Verification items for the finished model (mm, model axes). Coordinates: 2 decimals unless noted, no trailing zeros. Loops run counter-clockwise (first coordinate to the right, second up) from the corner with the lowest first, then second, coordinate; pieces in that order, holes last. Notation, with made-up numbers: (38.25, 11) - (50.25, 11) arc R21 ccw to (50.25, 23) - close; hole circle Ø1 at (-9.75, -19). An arc over 180 degrees is marked (long way). One line per item, written item: value. Start each with the question number.
(1) Section check A-A (x = -1.5). Record the boundary of the cut face in (y, z), plus the area to 3 significant figures.
(2) Thickness scan on probe 1 along X at (y, z) = (18, -39.85); probe 2 along X at (y, z) = (-31.5, -39.7); probe 3 along Y at (x, z) = (-14.5, -39.3). Record the ranges inside material, lowest first. Write a range as [from, to].
(3) Gauge pin test, flat end, axial feed: P1, Ø2, axis at x = 34.45, y = 5.84, coming from the -Z side. Record the tip position at first contact, or that the pin passes through.
(4) Section check B-B (x = 10). Record the boundary of the cut face in (y, z).
(5) Section check C-C (z = -40.35). Count the separate pieces of the cut face and the enclosed holes in it, plus the area to 3 significant figures.
(6) Draft check along Y on faces 1 (the face through (-45.8, 36.99, -39.93)), 2 (the face through (33.947, 36.589, -39.95)), 3 (the face through (-45.702, -37.605, -39.93)), 4 (the face through (34.62, -17.47, -39.95)). Enter one of: +Y half, -Y half, draft (parallel to the pull), parting line (faces both ways), or undercut.
```python
from build123d import *

# Parameters (mm, degrees)
EXTRUDE_1_DEPTH     = 1.5
SKETCH_3_R          = 1.3
CUT_EXTRUDE_1_DEPTH = 65.139634718
CUT_EXTRUDE_2_REACH = 66.14
SKETCH_4_R          = 1.3
CUT_EXTRUDE_3_REACH = 66.14
SKETCH_5_W          = 53
SKETCH_5_H          = 6.5
FILLET_1_R          = 1.5
CUT_EXTRUDE_4_REACH = 66.14
SKETCH_7_R          = 1.3
CUT_EXTRUDE_5_REACH = 66.14


with BuildPart() as part:
    # 草图2 → 凸台-拉伸1 (new body)
    with BuildSketch(Plane(origin=(0, 0, -39.19), x_dir=(-1, 0, 0), z_dir=(0, 0, -1))):
        Polygon((-47.34673203, -34.053824425), (-40.342568974, -41.057987481), (42.249104914, -41.057987481), (49.25326797, -34.053824425), (49.25326797, 33.537849463), (42.249104914, 40.542012519), (-40.342568974, 40.542012519), (-47.34673203, 33.537849463), align=None)
    extrude(amount=EXTRUDE_1_DEPTH)

    # 草图3 → 切除-拉伸1 (cut, through all)
    with BuildSketch(Plane(origin=(0, 0, -40.69), x_dir=(-1, 0, 0), z_dir=(0, 0, -1))):
        with Locations((-34.54673203, -38.257987481)):
            Circle(SKETCH_3_R)
        with Locations((36.45326797, -38.257987481)):
            Circle(SKETCH_3_R)
        with Locations((-34.54673203, 37.742012519)):
            Circle(SKETCH_3_R)
        with Locations((36.45326797, 37.742012519)):
            Circle(SKETCH_3_R)
    extrude(amount=-CUT_EXTRUDE_1_DEPTH, mode=Mode.SUBTRACT)

    # 草图4 → 切除-拉伸2 (cut, up to next)
    with BuildSketch(Plane(origin=(0, 0, -40.69), x_dir=(-1, 0, 0), z_dir=(0, 0, -1)), mode=Mode.PRIVATE) as cut_extrude_2_sk1:
        with Locations((23.45326797, -31.293200074)):
            Circle(SKETCH_4_R)
    cut_extrude_2_tool1 = extrude(cut_extrude_2_sk1.sketch, amount=-CUT_EXTRUDE_2_REACH, mode=Mode.PRIVATE) & part.part
    # 草图4 → 切除-拉伸2 (cut, up to next)
    with BuildSketch(Plane(origin=(0, 0, -40.69), x_dir=(-1, 0, 0), z_dir=(0, 0, -1)), mode=Mode.PRIVATE) as cut_extrude_2_sk2:
        with Locations((-34.558299802, -31.293200074)):
            Circle(SKETCH_4_R)
    cut_extrude_2_tool2 = extrude(cut_extrude_2_sk2.sketch, amount=-CUT_EXTRUDE_2_REACH, mode=Mode.PRIVATE) & part.part
    # 草图4 → 切除-拉伸2 (cut, up to next)
    with BuildSketch(Plane(origin=(0, 0, -40.69), x_dir=(-1, 0, 0), z_dir=(0, 0, -1)), mode=Mode.PRIVATE) as cut_extrude_2_sk3:
        with Locations((23.45326797, 17.742012519)):
            Circle(SKETCH_4_R)
    cut_extrude_2_tool3 = extrude(cut_extrude_2_sk3.sketch, amount=-CUT_EXTRUDE_2_REACH, mode=Mode.PRIVATE) & part.part
    # 草图4 → 切除-拉伸2 (cut, up to next)
    with BuildSketch(Plane(origin=(0, 0, -40.69), x_dir=(-1, 0, 0), z_dir=(0, 0, -1)), mode=Mode.PRIVATE) as cut_extrude_2_sk4:
        with Locations((-34.558299802, 17.742012519)):
            Circle(SKETCH_4_R)
    cut_extrude_2_tool4 = extrude(cut_extrude_2_sk4.sketch, amount=-CUT_EXTRUDE_2_REACH, mode=Mode.PRIVATE) & part.part
    add(cut_extrude_2_tool1.solids().sort_by_distance((-23.453268, -31.2932, -40.69))[0], mode=Mode.SUBTRACT)
    add(cut_extrude_2_tool2.solids().sort_by_distance((34.5583, -31.2932, -40.69))[0], mode=Mode.SUBTRACT)
    add(cut_extrude_2_tool3.solids().sort_by_distance((-23.453268, 17.742013, -40.69))[0], mode=Mode.SUBTRACT)
    add(cut_extrude_2_tool4.solids().sort_by_distance((34.5583, 17.742013, -40.69))[0], mode=Mode.SUBTRACT)

    # 草图5 → 切除-拉伸3 (cut, up to next)
    with BuildSketch(Plane(origin=(0, 0, -40.69), x_dir=(-1, 0, 0), z_dir=(0, 0, -1)), mode=Mode.PRIVATE) as cut_extrude_3_sk1:
        with Locations((-5.64673203, 17.992012519)):
            Rectangle(SKETCH_5_W, SKETCH_5_H)
    cut_extrude_3_tool1 = extrude(cut_extrude_3_sk1.sketch, amount=-CUT_EXTRUDE_3_REACH, mode=Mode.PRIVATE) & part.part
    add(cut_extrude_3_tool1.solids().sort_by_distance((5.646732, 17.992013, -40.69))[0], mode=Mode.SUBTRACT)

    # 圆角1
    fillet_1_edges = [part.edges().sort_by_distance(p)[0] for p in [
        (32.14673203, 14.742012519, -39.94),
        (32.14673203, 21.242012519, -39.94),
        (-20.85326797, 21.242012519, -39.94),
        (-20.85326797, 14.742012519, -39.94),
    ]]
    fillet(fillet_1_edges, radius=FILLET_1_R)

    # 草图7 → 切除-拉伸4 (cut, up to next)
    with BuildSketch(Plane(origin=(0, 0, -40.69), x_dir=(-1, 0, 0), z_dir=(0, 0, -1)), mode=Mode.PRIVATE) as cut_extrude_4_sk1:
        with Locations((-34.44673203, 5.842012519)):
            Circle(SKETCH_7_R)
    cut_extrude_4_tool1 = extrude(cut_extrude_4_sk1.sketch, amount=-CUT_EXTRUDE_4_REACH, mode=Mode.PRIVATE) & part.part
    # 草图7 → 切除-拉伸4 (cut, up to next)
    with BuildSketch(Plane(origin=(0, 0, -40.69), x_dir=(-1, 0, 0), z_dir=(0, 0, -1)), mode=Mode.PRIVATE) as cut_extrude_4_sk2:
        with Locations((-34.44673203, -18.757987481)):
            Circle(SKETCH_7_R)
    cut_extrude_4_tool2 = extrude(cut_extrude_4_sk2.sketch, amount=-CUT_EXTRUDE_4_REACH, mode=Mode.PRIVATE) & part.part
    # 草图7 → 切除-拉伸4 (cut, up to next)
    with BuildSketch(Plane(origin=(0, 0, -40.69), x_dir=(-1, 0, 0), z_dir=(0, 0, -1)), mode=Mode.PRIVATE) as cut_extrude_4_sk3:
        with Locations((-9.84673203, 5.842012519)):
            Circle(SKETCH_7_R)
    cut_extrude_4_tool3 = extrude(cut_extrude_4_sk3.sketch, amount=-CUT_EXTRUDE_4_REACH, mode=Mode.PRIVATE) & part.part
    # 草图7 → 切除-拉伸4 (cut, up to next)
    with BuildSketch(Plane(origin=(0, 0, -40.69), x_dir=(-1, 0, 0), z_dir=(0, 0, -1)), mode=Mode.PRIVATE) as cut_extrude_4_sk4:
        with Locations((-9.84673203, -18.757987481)):
            Circle(SKETCH_7_R)
    cut_extrude_4_tool4 = extrude(cut_extrude_4_sk4.sketch, amount=-CUT_EXTRUDE_4_REACH, mode=Mode.PRIVATE) & part.part
    add(cut_extrude_4_tool1.solids().sort_by_distance((34.446732, 5.842013, -40.69))[0], mode=Mode.SUBTRACT)
    add(cut_extrude_4_tool2.solids().sort_by_distance((34.446732, -18.757987, -40.69))[0], mode=Mode.SUBTRACT)
    add(cut_extrude_4_tool3.solids().sort_by_distance((9.846732, 5.842013, -40.69))[0], mode=Mode.SUBTRACT)
    add(cut_extrude_4_tool4.solids().sort_by_distance((9.846732, -18.757987, -40.69))[0], mode=Mode.SUBTRACT)

    # 草图8 → 切除-拉伸5 (cut, up to next)
    with BuildSketch(Plane(origin=(0, 0, -40.69), x_dir=(-1, 0, 0), z_dir=(0, 0, -1)), mode=Mode.PRIVATE) as cut_extrude_5_sk1:
        with BuildLine():
            Line((-29.92124863, 3.862113532), (-11.826631017, -14.232504081))
            ThreePointArc((-11.826631017, -14.232504081), (-11.826631017, -16.778088493), (-14.372215429, -16.778088493))
            Line((-14.372215429, -16.778088493), (-32.466833042, 1.31652912))
            ThreePointArc((-32.466833042, 1.31652912), (-32.466833042, 3.862113532), (-29.92124863, 3.862113532))
        make_face()
    cut_extrude_5_tool1 = extrude(cut_extrude_5_sk1.sketch, amount=-CUT_EXTRUDE_5_REACH, mode=Mode.PRIVATE) & part.part
    # 草图8 → 切除-拉伸5 (cut, up to next)
    with BuildSketch(Plane(origin=(0, 0, -40.69), x_dir=(-1, 0, 0), z_dir=(0, 0, -1)), mode=Mode.PRIVATE) as cut_extrude_5_sk2:
        with BuildLine():
            Line((-33.173939824, -1.485195275), (-17.173939824, -17.485195275))
            ThreePointArc((-17.173939824, -17.485195275), (-17.173939824, -20.030779687), (-19.719524236, -20.030779687))
            Line((-19.719524236, -20.030779687), (-35.719524236, -4.030779687))
            ThreePointArc((-35.719524236, -4.030779687), (-35.719524236, -1.485195275), (-33.173939824, -1.485195275))
        make_face()
    cut_extrude_5_tool2 = extrude(cut_extrude_5_sk2.sketch, amount=-CUT_EXTRUDE_5_REACH, mode=Mode.PRIVATE) & part.part
    # 草图8 → 切除-拉伸5 (cut, up to next)
    with BuildSketch(Plane(origin=(0, 0, -40.69), x_dir=(-1, 0, 0), z_dir=(0, 0, -1)), mode=Mode.PRIVATE) as cut_extrude_5_sk3:
        with BuildLine():
            Line((-24.573939824, 7.114804725), (-8.573939824, -8.885195275))
            ThreePointArc((-8.573939824, -8.885195275), (-8.573939824, -11.430779687), (-11.119524236, -11.430779687))
            Line((-11.119524236, -11.430779687), (-27.119524236, 4.569220313))
            ThreePointArc((-27.119524236, 4.569220313), (-27.119524236, 7.114804725), (-24.573939824, 7.114804725))
        make_face()
    cut_extrude_5_tool3 = extrude(cut_extrude_5_sk3.sketch, amount=-CUT_EXTRUDE_5_REACH, mode=Mode.PRIVATE) & part.part
    # 草图8 → 切除-拉伸5 (cut, up to next)
    with BuildSketch(Plane(origin=(0, 0, -40.69), x_dir=(-1, 0, 0), z_dir=(0, 0, -1)), mode=Mode.PRIVATE) as cut_extrude_5_sk4:
        with BuildLine():
            Line((-16.573939824, 7.114804725), (-8.573939824, -0.885195275))
            ThreePointArc((-8.573939824, -0.885195275), (-8.573939824, -3.430779687), (-11.119524236, -3.430779687))
            Line((-11.119524236, -3.430779687), (-19.119524236, 4.569220313))
            ThreePointArc((-19.119524236, 4.569220313), (-19.119524236, 7.114804725), (-16.573939824, 7.114804725))
        make_face()
    cut_extrude_5_tool4 = extrude(cut_extrude_5_sk4.sketch, amount=-CUT_EXTRUDE_5_REACH, mode=Mode.PRIVATE) & part.part
    # 草图8 → 切除-拉伸5 (cut, up to next)
    with BuildSketch(Plane(origin=(0, 0, -40.69), x_dir=(-1, 0, 0), z_dir=(0, 0, -1)), mode=Mode.PRIVATE) as cut_extrude_5_sk5:
        with BuildLine():
            Line((-33.173939824, -9.485195275), (-25.173939824, -17.485195275))
            ThreePointArc((-25.173939824, -17.485195275), (-25.173939824, -20.030779687), (-27.719524236, -20.030779687))
            Line((-27.719524236, -20.030779687), (-35.719524236, -12.030779687))
            ThreePointArc((-35.719524236, -12.030779687), (-35.719524236, -9.485195275), (-33.173939824, -9.485195275))
        make_face()
    cut_extrude_5_tool5 = extrude(cut_extrude_5_sk5.sketch, amount=-CUT_EXTRUDE_5_REACH, mode=Mode.PRIVATE) & part.part
    add(cut_extrude_5_tool1.solids().sort_by_distance((22.146732, -6.457987, -40.69))[0], mode=Mode.SUBTRACT)
    add(cut_extrude_5_tool2.solids().sort_by_distance((26.446732, -10.757987, -40.69))[0], mode=Mode.SUBTRACT)
    add(cut_extrude_5_tool3.solids().sort_by_distance((17.846732, -2.157987, -40.69))[0], mode=Mode.SUBTRACT)
    add(cut_extrude_5_tool4.solids().sort_by_distance((13.846732, 1.842013, -40.69))[0], mode=Mode.SUBTRACT)
    add(cut_extrude_5_tool5.solids().sort_by_distance((30.446732, -14.757987, -40.69))[0], mode=Mode.SUBTRACT)


solid = part.part
```
Responses:
1. outline: (-41.06, -40.69) - (14.74, -40.69) - (14.74, -39.19) - (-41.06, -39.19) - close; (21.24, -40.69) - (40.54, -40.69) - (40.54, -39.19) - (21.24, -39.19) - close
1. area: 113 mm²
2. probe 1: x = [-49.25, -24.73], [-22.18, -20.85], [32.15, 33.28], [35.83, 47.35]
2. probe 2: x = [-49.25, -24.74], [-22.17, 33.27], [35.84, 47.35]
2. probe 3: y = [-41.06, 14.74], [21.24, 40.54]
3. P1: passes through
4. outline: (-41.06, -40.69) - (-20.05, -40.69) - (-20.05, -39.19) - (-41.06, -39.19) - close; (-17.47, -40.69) - (-11.95, -40.69) - (-11.95, -39.19) - (-17.47, -39.19) - close; (-7.46, -40.69) - (-3.95, -40.69) - (-3.95, -39.19) - (-7.46, -39.19) - close; (0.54, -40.69) - (4.55, -40.69) - (4.55, -39.19) - (0.54, -39.19) - close; (7.13, -40.69) - (14.74, -40.69) - (14.74, -39.19) - (7.13, -39.19) - close; (21.24, -40.69) - (40.54, -40.69) - (40.54, -39.19) - (21.24, -39.19) - close
5. separate pieces: 1
5. enclosed holes: 18
5. area: 6,990 mm²
6. face 1: +Y half
6. face 2: undercut
6. face 3: -Y half
6. face 4: undercut
